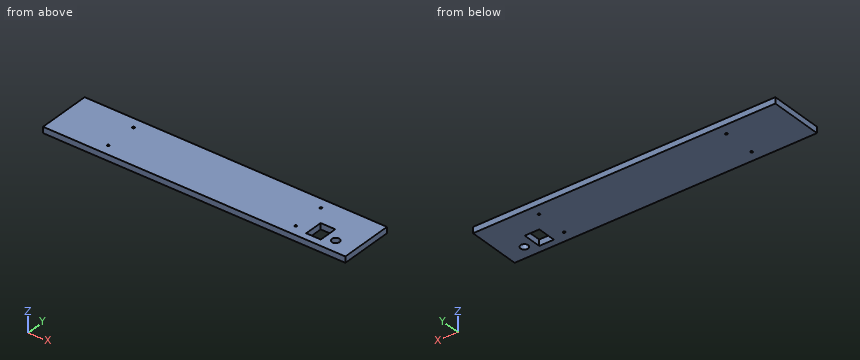
```python
from build123d import *

# Parameters (mm, degrees)
SZKIC1_W                    = 451
SZKIC1_H                    = 80
DODANIE_WYCI_GNI_CIE1_DEPTH = 9
SZKIC2_W                    = 21.8
SZKIC2_H                    = 27.7
SZKIC2_R                    = 5.75
SZKIC2_R_2                  = 1.65
WYTNIJ_WYCI_GNI_CIE1_DEPTH  = 10


with BuildPart() as part:
    # Szkic1 → Dodanie-wyciągnięcie1 (new body)
    with BuildSketch(Plane.XY):
        with Locations((225.5, 40)):
            Rectangle(SZKIC1_W, SZKIC1_H)
    extrude(amount=-DODANIE_WYCI_GNI_CIE1_DEPTH)

    # Szkic2 → Wytnij-wyciągnięcie1 (cut)
    with BuildSketch(Plane.XY):
        with Locations((395.1, 24.64)):
            Rectangle(SZKIC2_W, SZKIC2_H)
        with Locations((421, 20)):
            Circle(SZKIC2_R)
        with Locations((364.78, 64.21)):
            Circle(SZKIC2_R_2)
        with Locations((364.78, 15.79)):
            Circle(SZKIC2_R_2)
        with Locations((85.22, 64.21)):
            Circle(SZKIC2_R_2)
        with Locations((85.22, 15.79)):
            Circle(SZKIC2_R_2)
    extrude(amount=-WYTNIJ_WYCI_GNI_CIE1_DEPTH, mode=Mode.SUBTRACT)


solid = part.part
```
Verification items for the finished model (mm, model axes). Round coordinates to 2 decimals unless told otherwise and drop trailing zeros. Write each loop counter-clockwise with the first axis right and the second up, starting at its lowest first coordinate (ties: lowest second). Pieces come first, ordered by that corner, then holes. Notation, with made-up numbers: (43, 59) -> (90, 59) arc R5 ccw to (90, 65) -> close; hole circle Ø9 at (30, 39.5). An arc over 180 degrees is marked (long way). Write each question's results on one line, items separated by ' | '. Start each with the question number.
1. Material ranges on probe 1 along Y at (x, z) = (85.5, -6.5); probe 2 along Y at (x, z) = (364.78, -4.75); probe 3 along X at (y, z) = (64.5, -1.5), recorded low to high. Write a range as from..to.
2. Cross-section at B-B (z = -6.25). Enter the section's corners in (x, y).
3. Depth check by flat-ended pin: P1, Ø10.5, axis at x = 421, y = 20, coming from the -Z side. Enter the tip coordinate at first touch or a pass-through.
4. Cross-section at A-A (x = 421). Enter the section's corners in (y, z).
Solutions:
1) probe 1: y = 0..14.16, 17.42..62.58, 65.84..80 | probe 2: y = 0..14.14, 17.44..62.56, 65.86..80 | probe 3: x = 0..83.6, 86.84..363.16, 366.4..451
2) outline: (0, 0) -> (451, 0) -> (451, 80) -> (0, 80) -> close; hole circle Ø3.3 at (85.22, 15.79); hole circle Ø3.3 at (85.22, 64.21); hole circle Ø3.3 at (364.78, 15.79); hole circle Ø3.3 at (364.78, 64.21); hole (384.2, 10.79) -> (406, 10.79) -> (406, 38.49) -> (384.2, 38.49) -> close; hole circle Ø11.5 at (421, 20)
3) P1: passes through
4) outline: (0, -9) -> (14.25, -9) -> (14.25, 0) -> (0, 0) -> close; (25.75, -9) -> (80, -9) -> (80, 0) -> (25.75, 0) -> close
